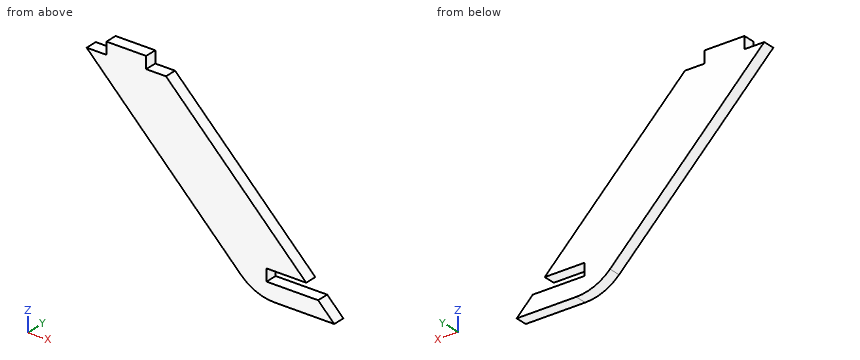
from build123d import *

# Parameters (mm, degrees)
RESSALTO_EXTRUS_O1_DEPTH = 3


with BuildPart() as part:
    # Esboço1 → Ressalto-extrusão1 (new body)
    with BuildSketch(Plane(origin=(0, 0, 0), x_dir=(1, 0, 0), z_dir=(0, 1, 0))):
        with BuildLine():
            Line((-12.989253032, -17.540319489), (-2.989253032, -17.540319489))
            Line((-2.989253032, -17.540319489), (-2.989253032, -14.540319489))
            Line((-2.989253032, -14.540319489), (2.010746968, -14.540319489))
            Line((2.010746968, -14.540319489), (37.366086027, 20.81501957))
            Line((37.366086027, 20.81501957), (27.366086027, 20.81501957))
            Line((27.366086027, 20.81501957), (27.366086027, 23.81501957))
            Line((27.366086027, 23.81501957), (40.366086027, 23.81501957))
            Line((40.366086027, 23.81501957), (44.437153839, 27.886087382))
            Line((44.437153839, 27.886087382), (29.437153839, 27.886087382))
            ThreePointArc((29.437153839, 27.886087382), (24.817756177, 26.967232057), (20.901619933, 24.350553476))
            Line((20.901619933, 24.350553476), (-17.989253032, -14.540319489))
            Line((-17.989253032, -14.540319489), (-12.989253032, -14.540319489))
            Line((-12.989253032, -14.540319489), (-12.989253032, -17.540319489))
        make_face()
    extrude(amount=RESSALTO_EXTRUS_O1_DEPTH)


solid = part.part
Verification items for the finished model (mm, model axes). Coordinates: 2 decimals unless noted, no trailing zeros. Loops run counter-clockwise (first coordinate to the right, second up) from the corner with the lowest first, then second, coordinate; pieces in that order, holes last. Notation, with made-up numbers: M 82.25,-10.75 L 129.25,-10.75 A34 ccw 129.25,26.25 Z; hole C 66.5,-6 d6. An arc over 180 degrees is marked long. One line per item, written item: value.
1. Section check A-A on x = 35. Record the cut outline in (y, z).
Answers follow:
outline: M 0,-27.89 L 3,-27.89 L 3,-23.82 L 0,-23.82 Z; M 0,-20.82 L 3,-20.82 L 3,-18.45 L 0,-18.45 Z
2. Gauge pin test, flat ends, axial feed: P1, Ø1.5, axis at y = 1.5, z = -1.5, coming from the +X side; P2, Ø1.5, axis at x = -1, y = 1, coming from the +Z side; P3, Ø1, axis at y = 1.5, z = -11.5, coming from the +X side. Record the tip position at first contact, or that the pin passes through.
Answers follow:
P1: x = 18.8
P2: z = 14.54
P3: x = 28.55
3. Section check C-C on z = -22. Record the cut outline in (x, y), plus the area to 3 significant figures.
Answers follow:
outline: M 18.55,0 L 27.37,0 L 27.37,3 L 18.55,3 Z
area: 26.4 mm^2
4. Material ranges on line 1 along Z through (x, y) = (32.5, 1.3); line 2 along Z through (x, y) = (37.5, 0.75); line 3 along X through (y, z) = (1.3, -15), recorded low to high. Write a range as from..to.
Answers follow:
line 1: -27.89..-23.82, -20.82..-15.95
line 2: -27.89..-23.82
line 3: 11.55..31.55
5. Section check B-B on y = 1.4. Record the cut outline in (x, z).
Answers follow:
outline: M -17.99,14.54 L 20.9,-24.35 A12.07 ccw 29.44,-27.89 L 44.44,-27.89 L 40.37,-23.82 L 27.37,-23.82 L 27.37,-20.82 L 37.37,-20.82 L 2.01,14.54 L -2.99,14.54 L -2.99,17.54 L -12.99,17.54 L -12.99,14.54 Z
6. Section check D-D on x = 25.5. Record the cut outline in (y, z), plus the area to 3 significant figures.
Answers follow:
outline: M 0,-27.23 L 3,-27.23 L 3,-8.95 L 0,-8.95 Z
area: 54.8 mm^2
